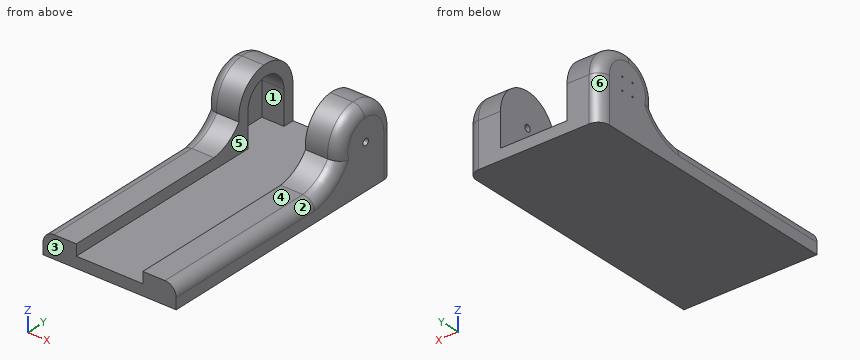
Autodesk Inventor part; units mm, degrees
ref_plane "Work Plane1" through (0, -300, 0) normal (1, 0, 0) x (0, 0, -1)
ref_plane "YZ Plane" through (0, 0, 0) normal (1, 0, 0) x (0, 1, 0)
ref_plane "XZ Plane" through (0, 0, 0) normal (0, 1, 0) x (-1, 0, 0)
sketch "Sketch1" plane through (0, 0, 0) normal (0, 0, 1) x (1, 0, 0)
  line L0 (-150, -300) -> (150, -300)
  line L1 (150, -300) -> (150, 300)
  line L2 (150, 300) -> (-150, 300)
  line L3 (-150, 300) -> (-150, -300)
  line L4 (-150, -300) -> (150, 300) construction
  line L5 (150, -300) -> (-150, 300) construction
  point P0 (0, 0)
  point P1 (0, 0)
  dimension "d23" = 300
  dimension "d24" = 600
sketch "Sketch1 outline for Extrusion1" plane through (0, 0, 0) normal (0, 0, 1) x (1, 0, 0)
  line L0 (-150, 300) -> (-150, -300)
  line L1 (150, 300) -> (-150, 300)
  line L2 (150, -300) -> (150, 300)
  line L3 (-150, -300) -> (150, -300)
extrude "Extrusion1" add sketch "Sketch1 outline for Extrusion1" along normal blind 25
sketch "Sketch15" plane through (-150, -300, 0) normal (-1, 0, 0) x (0, 0, 1)
  line L0 (0, 0) -> (0, 600) construction
  line L1 (0, 600) -> (300, 600) construction
  line L2 (0, 600) -> (300, 600) construction
  line L3 (25, 600) -> (25, 0) construction
  line L4 (0, 600) -> (25, 600)
  line L5 (25, 600) -> (100, 600)
  line L6 (25, 381.543819) -> (50, 381.543819) construction
  line L7 (25, 0) -> (50, 0)
  line L8 (50, 0) -> (50, 381.543819)
  arc A0 (174.804436, 519.587383) -> (100, 600) centre (100, 525) ccw
  arc A1 (90.513255, 450.602408) -> (174.804436, 519.587383) centre (100, 525) ccw
  arc A2 (90.513255, 450.602408) -> (50, 381.543819) centre (149.296649, 369.704246) ccw
  line L9 (25, 0) -> (25, 600)
  line L10 (25, 0) -> (25, 600)
  point P0 (0, 300)
  dimension "d54" = 300
  dimension "d55" = 0
  dimension "d59" = 25
  dimension "d60" = 25
  dimension "d61" = 75
  dimension "d62" = 75
  dimension "d63" = 75
  dimension "d65" = 100
  dimension "d79" = 124.29665
sketch "Sketch15 outline for Extrusion14" plane through (-150, -300, 0) normal (-1, 0, 0) x (0, 0, 1)
  line L0 (100, 600) -> (25, 600)
  arc A0 (174.804436, 519.587383) -> (100, 600) centre (100, 525) ccw
  arc A1 (90.513255, 450.602408) -> (174.804436, 519.587383) centre (100, 525) ccw
  arc A2 (50, 381.543819) -> (90.513255, 450.602408) centre (149.296649, 369.704246) cw
  line L1 (50, 0) -> (50, 381.543819)
  line L2 (25, 0) -> (50, 0)
  line L3 (25, 600) -> (25, 0)
extrude "Extrusion14" add sketch "Sketch15 outline for Extrusion14" against normal blind 300
ref_plane "Work Plane1" through (0, -300, 0) normal (1, 0, 0) x (0, 0, -1)
sketch "Sketch16" plane through (0, -300, 0) normal (1, 0, 0) x (0, 0, -1)
  line L0 (-175, 600) -> (-25, 600)
  line L1 (-25, 600) -> (-25, 0)
  line L2 (-25, 0) -> (-175, 0)
  line L3 (-175, 0) -> (-175, 600)
  point P0 (0, 300)
  dimension "d73" = 150
  dimension "d74" = 600
  dimension "d75" = 25
  dimension "d76" = 300
sketch "Sketch16 outline for Extrusion16" plane through (0, -300, 0) normal (1, 0, 0) x (0, 0, -1)
  line L0 (-175, 600) -> (-25, 600)
  line L1 (-25, 600) -> (-25, 0)
  line L2 (-25, 0) -> (-175, 0)
  line L3 (-175, 0) -> (-175, 600)
extrude "Extrusion16" cut sketch "Sketch16 outline for Extrusion16" along normal mid plane 150
sketch "Sketch17" plane through (-75, -300, 0) normal (1, 0, 0) x (0, 0, -1)
  arc A0 (-100, 600) -> (-90.513255, 450.602408) centre (-100, 525) ccw
  line L0 (-100, 475) -> (-25, 475)
  line L1 (-25, 475) -> (-25, 575)
  line L2 (-25, 575) -> (-100, 575)
  arc A1 (-100, 575) -> (-100, 475) centre (-100, 525) ccw
  line L3 (0, 600) -> (0, 0)
  point P0 (0, 300)
  dimension "d86" = 50
  dimension "d87" = 25
  dimension "d88" = 90
sketch "Sketch17 outline for Extrusion17" plane through (-75, -300, 0) normal (1, 0, 0) x (0, 0, -1)
  arc A0 (-100, 575) -> (-100, 475) centre (-100, 525) ccw
  line L0 (-25, 575) -> (-100, 575)
  line L1 (-25, 475) -> (-25, 575)
  line L2 (-100, 475) -> (-25, 475)
extrude "Extrusion17" cut sketch "Sketch17 outline for Extrusion17" against normal blind 50
sketch "Sketch21" plane through (-150, -300, 0) normal (-1, 0, 0) x (0, 0, 1)
  arc A0 (90.513255, 450.602408) -> (100, 600) centre (100, 525) ccw
  line L0 (85.857864, 510.857864) -> (114.142136, 510.857864) construction
  line L1 (114.142136, 510.857864) -> (114.142136, 539.142136) construction
  line L2 (114.142136, 539.142136) -> (85.857864, 539.142136) construction
  line L3 (85.857864, 539.142136) -> (85.857864, 510.857864) construction
  line L4 (114.142136, 510.857864) -> (85.857864, 539.142136) construction
  circle A1 centre (114.142136, 539.142136) radius 1.65
  circle A2 centre (85.857864, 539.142136) radius 1.65
  circle A3 centre (114.142136, 510.857864) radius 1.65
  circle A4 centre (85.857864, 510.857864) radius 1.65
  line L5 (85.857864, 510.857864) -> (114.142136, 539.142136) construction
  line L6 (0, 600) -> (0, 0) construction
  line L7 (0, 600) -> (100, 600)
  point P0 (0, 300)
  dimension "d102" = 28.28427
  dimension "d103" = 28.28427
  dimension "d104" = 3.3
  dimension "d105" = 3.3
  dimension "d106" = 3.3
  dimension "d107" = 3.3
  dimension "d111" = 85.85786
  dimension "d112" = 60.85786
sketch "Sketch21 outline for Extrusion21" plane through (-150, -300, 0) normal (-1, 0, 0) x (0, 0, 1)
  circle A0 centre (114.142136, 539.142136) radius 1.65
  circle A1 centre (85.857864, 539.142136) radius 1.65
  circle A2 centre (114.142136, 510.857864) radius 1.65
  circle A3 centre (85.857864, 510.857864) radius 1.65
extrude "Extrusion21" cut sketch "Sketch21 outline for Extrusion21" against normal blind 75
sketch "Sketch22" plane through (150, -300, 0) normal (1, 0, 0) x (0, 0, -1)
  circle A0 centre (-100, 525) radius 7.5
  arc A1 (-100, 600) -> (-90.513255, 450.602408) centre (-100, 525) ccw
  point P0 (0, 300)
  dimension "d113" = 15
sketch "Sketch22 outline for Extrusion22" plane through (150, -300, 0) normal (1, 0, 0) x (0, 0, -1)
  circle A0 centre (-100, 525) radius 7.5
extrude "Extrusion22" cut sketch "Sketch22 outline for Extrusion22" against normal blind 75
fillet "Fillet3" radius 25 8 edges at (-150, 300, 50) (-150, 220.2471, 174.8492) (-150, 120.3047, 63.0435) (-150, -109.2281, 50) (150, 300, 50) (150, 220.2471, 174.8492) (150, 120.3047, 63.0435) (150, -109.2281, 50)
properties material "ABS Plastic"
Geometry check sheet. Reference: the model listing, model coordinates, mm. Face numbers are marked on the shaded views. A direction names the side the tool comes from. Round coordinates to 2 decimals unless told otherwise and drop trailing zeros. Loops run counter-clockwise (first coordinate to the right, second up) from the corner with the lowest first, then second, coordinate; pieces in that order, holes last. Notation, with made-up numbers: (-19, 18) - (11, 18) arc R14 cw to (11, 29) - close; hole circle Ø1 at (40, -32.75). An arc over 180 degrees is marked (long way). Write each question's results on one line, items separated by ' | '. Start each with the question number.
Q1. Cross-section at A-A on x = -96. Enter the section's corners in (y, z).
Q2. Thickness scan on line 1 (Y direction, x = 93, z = 100); line 2 (X direction, y = 258, z = 55); line 3 (Z direction, x = 54, y = -226.5). Record the ranges inside material, lowest first. Write a range as [from, to].
Q3. Release check for a two-part mould opening along X. For the marked faces 1, 2 and 3 record: +X half, -X half, draft (parallel to the pull), parting line (faces both ways), or undercut.
Q4. Cross-section at B-B on x = 108. Enter the section's corners in (y, z).
Q5. Access from +Z, -Z, +X, -X, +Y, -Y to the whole of each face (thin tool, end or side, straight path). Record for the marked faces 4, 5 and 6.
Q6. Cross-section at C-C on x = 46.5. Enter the section's corners in (y, z).
Q7. Gauge pin test, flat ends, axial feed: P1, Ø25, axis at x = -89, y = -189, coming from the +Z side; P2, Ø2, axis at x = 53.5, y = 127, coming from the +Z side; P3, Ø10, axis at x = 67.5, z = 57, coming from the +Y side; P4, Ø12, axis at x = 106, z = 145, coming from the -Y side. Record the tip position at first contact, or that the pin passes through.
Answers below:
1) outline: (-300, 0) - (300, 0) - (300, 100) arc R75 ccw (long way) to (150.6, 90.51) arc R100 cw to (81.54, 50) - (-300, 50) - close; hole (175, 25) - (275, 25) - (275, 100) arc R50 ccw to (175, 100) - close
2) line 1: y = [150, 217.5], [232.5, 300] | line 2: x = [-150, -125], [75, 150] | line 3: z = [0, 25]
3) face 1: undercut | face 2: +X half | face 3: draft
4) outline: (-300, 0) - (300, 0) - (300, 100) arc R75 ccw (long way) to (150.6, 90.51) arc R100 cw to (81.54, 50) - (-300, 50) - close; hole circle Ø15 at (225, 100)
5) face 4: +Z, +X, -X, -Y | face 5: +Z, +Y, -Y | face 6: +Z, -Z, -X, +Y
6) outline: (-300, 0) - (300, 0) - (300, 25) - (-300, 25) - close
7) P1: stops at z = 50 | P2: stops at z = 25 | P3: passes through | P4: stops at y = 160.94
